from build123d import *

# Parameters (mm, degrees)
BOSS_EXTRUDE1_DEPTH = 15
SKETCH3_W           = 8.5
SKETCH3_H           = 16.5
SKETCH3_R           = 1
SKETCH3_R_2         = 1.5
BOSS_EXTRUDE2_DEPTH = 2
SKETCH4_W           = 6
SKETCH4_H           = 20
CUT_EXTRUDE1_DEPTH  = 2


with BuildPart() as part:
    # Sketch2 → Boss-Extrude1 (new body)
    with BuildSketch(Plane(origin=(0, 0, 0), x_dir=(1, 0, 0), z_dir=(0, 1, 0))):
        Polygon((0, 0), (-4.5, 0), (-4.5, -12.5), (0, -12.5), (0, -10.5), (2, -10.5), (2, -14.5), (-6.5, -14.5), (-6.5, 2), (2, 2), (2, -2), (0, -2), align=None)
    extrude(amount=BOSS_EXTRUDE1_DEPTH)

    # Sketch3 → Boss-Extrude2 (add)
    with BuildSketch(Plane.XZ):
        with Locations((-2.25, 6.25)):
            Rectangle(SKETCH3_W, SKETCH3_H)
        with Locations((-3.5, 11.5)):
            Circle(SKETCH3_R, mode=Mode.SUBTRACT)
        with Locations((-3.5, 6.5)):
            Circle(SKETCH3_R_2, mode=Mode.SUBTRACT)
    extrude(amount=BOSS_EXTRUDE2_DEPTH)

    # Sketch4 → Cut-Extrude1 (cut)
    with BuildSketch(Plane(origin=(-4.5, 0, 0), x_dir=(0, 0, -1), z_dir=(1, 0, 0))):
        with Locations((-6.25, 10)):
            Rectangle(SKETCH4_W, SKETCH4_H)
    extrude(amount=-CUT_EXTRUDE1_DEPTH, mode=Mode.SUBTRACT)


solid = part.part
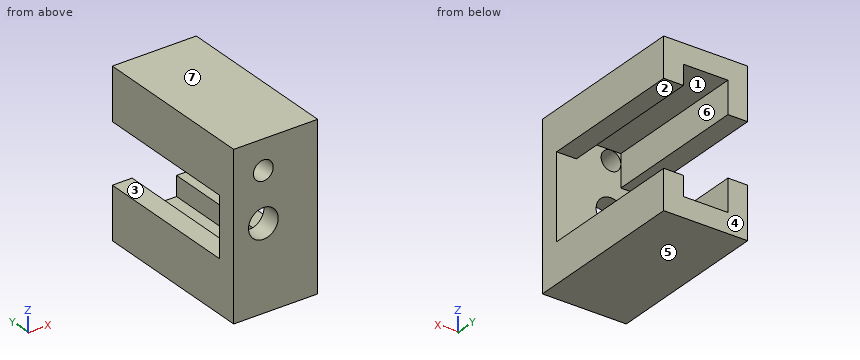
Part model, mm, in its own coordinate system. Face numbers are marked on the shaded views. A direction names the side the tool comes from. Round coordinates to 2 decimals unless told otherwise and drop trailing zeros. Order: outer loops, then holes, each group sorted by start corner. A loop starts at its lowest first (then second) coordinate and runs counter-clockwise, first axis right, second up. Notation, with made-up numbers: (20, -1) -> (32, -1) arc R18 ccw to (32, 13) -> close; hole circle Ø11 at (55.25, 89.5). An arc over 180 degrees is marked (long way). Put each result on its own line as item: value.
Q1. Band-saw the part on A-A (z = 6.5). Give the cut face in (x, y), and give its area (3 significant figures).
From the geometry:
outline: (-6.5, -2) -> (-5, -2) -> (-5, 0) -> (-6.5, 0) -> close; (-2, -2) -> (2, -2) -> (2, 0) -> (-2, 0) -> close
area: 11.0 mm2
Q2. Wall check: line 1 (Z direction, x = -3.5, y = -1.3); line 2 (X direction, y = 8.5, z = 1); line 3 (X direction, y = -0.75, z = 11.5). Give the ranges that are in metal, low to high. Write a range as [from, to].
From the geometry:
line 1: z = [-2, 5], [8, 10.5], [12.5, 14.5]
line 2: x = [-6.5, -4.5], [0, 2]
line 3: x = [-6.5, -4.5], [-2.5, 2]
Q3. Pull direction Z, two halves, no side cores. Call the marked faces 5, 6 and 7: pulls with the +Z half, pulls with the -Z half, needs draft (parallel to the pull), parting line crosses it, or undercut.
From the geometry:
face 5: pulls with the -Z half
face 6: undercut
face 7: pulls with the +Z half
Q4. Band-saw the part on D-D (y = -0.75). Give the cut face in (x, z).
From the geometry:
outline: (-6.5, -2) -> (2, -2) -> (2, 14.5) -> (-6.5, 14.5) -> close; hole circle Ø3 at (-3.5, 6.5); hole circle Ø2 at (-3.5, 11.5)
Q5. Tool access for the marked faces 1, 2, 3 and 4: list every direction of +Z, -Z, +X, -X, +Y, -Y with a clear straight run to the whole face (end or side of a thin tool).
From the geometry:
face 1: +Y
face 2: +X, +Y
face 3: +X, -X, +Y
face 4: +Z, -Z, +X, -X, +Y
Q6. Band-saw the part on B-B (y = 7.25). Give the cut face in (x, z).
From the geometry:
outline: (-6.5, -2) -> (2, -2) -> (2, 2) -> (0, 2) -> (0, 0) -> (-4.5, 0) -> (-4.5, 3.25) -> (-6.5, 3.25) -> close; (-6.5, 9.25) -> (-4.5, 9.25) -> (-4.5, 12.5) -> (0, 12.5) -> (0, 10.5) -> (2, 10.5) -> (2, 14.5) -> (-6.5, 14.5) -> close
Q7. Band-saw the part on C-C (x = -1). Give the cut face in (y, z).
From the geometry:
outline: (-2, -2) -> (15, -2) -> (15, 0) -> (0, 0) -> (0, 12.5) -> (15, 12.5) -> (15, 14.5) -> (-2, 14.5) -> close
Q8. Pin check, flat tips, straight feed: pin 1 Ø4 at (x, z) = (0, 6) entering from +Y; pin 2 Ø2.5 at (x, z) = (-3.5, 6.5) entering from +Y; pin 3 Ø2.5 at (x, z) = (-3.5, 11.5) entering from +Y. Stop position of each tip, or through.
From the geometry:
pin 1: stops at y = 0
pin 2: passes through
pin 3: stops at y = 15
